CAD build for the part. Positions are in the model's coordinates, mm. Face numbers are marked on the shaded views. A direction names the side the tool comes from. Give positions to 0.01 mm unless a question says otherwise; leave off trailing zeros. Loops run counter-clockwise (first coordinate to the right, second up) from the corner with the lowest first, then second, coordinate; pieces in that order, holes last. Notation, with made-up numbers: (67, 81) - (123, 81) arc R25 cw to (123, 105) - close; hole circle Ø7 at (32, -29). An arc over 180 degrees is marked (long way). Return JSON: item names as keys, results as strings.
from build123d import *

# Parameters (mm, degrees)
BOSS_EXTRUDE2_DEPTH = 80
SKETCH3_R           = 2
CUT_EXTRUDE2_DEPTH  = 80
SKETCH4_W           = 20
SKETCH4_H           = 80
BOSS_EXTRUDE3_DEPTH = 50
BOSS_EXTRUDE4_DEPTH = 80
SKETCH6_W           = 12
SKETCH6_H           = 60
CUT_EXTRUDE4_DEPTH  = 90
SKETCH7_W           = 3
SKETCH7_H           = 68
CUT_EXTRUDE5_DEPTH  = 90
SKETCH9_R           = 2
CUT_EXTRUDE6_DEPTH  = 90
SKETCH11_R          = 2
CUT_EXTRUDE7_DEPTH  = 90


with BuildPart() as part:
    # Sketch1 → Boss-Extrude2 (new body)
    with BuildSketch(Plane.XY):
        with BuildLine():
            ThreePointArc((26, -15.25), (25.707106781, -15.957106781), (25, -16.25))
            Line((25, -16.25), (-19, -16.25))
            Line((-19, -16.25), (-19, 16.25))
            Line((-19, 16.25), (4, 16.25))
            Line((4, 16.25), (53, 16.25))
            ThreePointArc((53, 16.25), (53.707106781, 15.957106781), (54, 15.25))
            Line((54, 15.25), (54, 10.25))
            Line((54, 10.25), (2, 10.25))
            ThreePointArc((2, 10.25), (0.585786438, 9.664213562), (0, 8.25))
            Line((0, 8.25), (0, -8.25))
            ThreePointArc((0, -8.25), (0.585786438, -9.664213562), (2, -10.25))
            Line((2, -10.25), (25, -10.25))
            ThreePointArc((25, -10.25), (25.707106781, -10.542893219), (26, -11.25))
            Line((26, -11.25), (26, -15.25))
        make_face()
    extrude(amount=BOSS_EXTRUDE2_DEPTH)

    # Sketch3 → Cut-Extrude2 (cut)
    with BuildSketch(Plane(origin=(0, 16.25, 0), x_dir=(1, 0, 0), z_dir=(0, 1, 0))):
        with Locations(Location((10.2, -40, 0), (0, 0, 270))):
            Circle(SKETCH3_R)
        with Locations(Location((10.2, -60, 0), (0, 0, 270))):
            Circle(SKETCH3_R)
        with Locations(Location((10.2, -20, 0), (0, 0, 270))):
            Circle(SKETCH3_R)
    extrude(amount=-CUT_EXTRUDE2_DEPTH, mode=Mode.SUBTRACT)

    # Sketch4 → Boss-Extrude3 (add)
    with BuildSketch(Plane(origin=(0, 16.25, 0), x_dir=(1, 0, 0), z_dir=(0, 1, 0))):
        with Locations((-9, -40)):
            Rectangle(SKETCH4_W, SKETCH4_H)
    extrude(amount=BOSS_EXTRUDE3_DEPTH)

    # Sketch5 → Boss-Extrude4 (add)
    with BuildSketch(Plane.XY.offset(80)):
        with BuildLine():
            ThreePointArc((4.354101966, 16.25), (2.2624519, 16.94375696), (1, 18.75))
            Line((1, 18.75), (1, 16.25))
            Line((1, 16.25), (4.354101966, 16.25))
        make_face()
    extrude(amount=-BOSS_EXTRUDE4_DEPTH)

    # Sketch6 → Cut-Extrude4 (cut)
    with BuildSketch(Plane(origin=(0, 66.25, 0), x_dir=(1, 0, 0), z_dir=(0, 1, 0))):
        with Locations((-13, -40)):
            Rectangle(SKETCH6_W, SKETCH6_H)
        with BuildLine():
            ThreePointArc((-17.5, -80), (-18.560660172, -79.560660172), (-19, -78.5))
            Line((-19, -78.5), (-19, -80))
            Line((-19, -80), (-17.5, -80))
        make_face()
        with BuildLine():
            Line((-19, 0), (-19, -1.5))
            ThreePointArc((-19, -1.5), (-18.560660172, -0.439339828), (-17.5, 0))
            Line((-17.5, 0), (-19, 0))
        make_face()
    extrude(amount=-CUT_EXTRUDE4_DEPTH, mode=Mode.SUBTRACT)

    # Sketch7 → Cut-Extrude5 (cut)
    with BuildSketch(Plane(origin=(0, 66.25, 0), x_dir=(1, 0, 0), z_dir=(0, 1, 0))):
        with Locations((-8.5, -40)):
            Rectangle(SKETCH7_W, SKETCH7_H)
    extrude(amount=-CUT_EXTRUDE5_DEPTH, mode=Mode.SUBTRACT)

    # Sketch9 → Cut-Extrude6 (cut)
    with BuildSketch(Plane(origin=(1, 0, 0), x_dir=(0, 0, -1), z_dir=(1, 0, 0))):
        with Locations(Location((-49.9, 36.25, 0), (0, 0, 90))):
            Circle(SKETCH9_R)
        with Locations(Location((-30.1, 36.25, 0), (0, 0, 90))):
            Circle(SKETCH9_R)
    extrude(amount=-CUT_EXTRUDE6_DEPTH, mode=Mode.SUBTRACT)

    # Sketch11 → Cut-Extrude7 (cut)
    with BuildSketch(Plane(origin=(1, 0, 0), x_dir=(0, 0, -1), z_dir=(1, 0, 0))):
        with Locations(Location((-40, 36.25, 0), (0, 0, 90))):
            Circle(SKETCH11_R)
    extrude(amount=-CUT_EXTRUDE7_DEPTH, mode=Mode.SUBTRACT)


solid = part.part
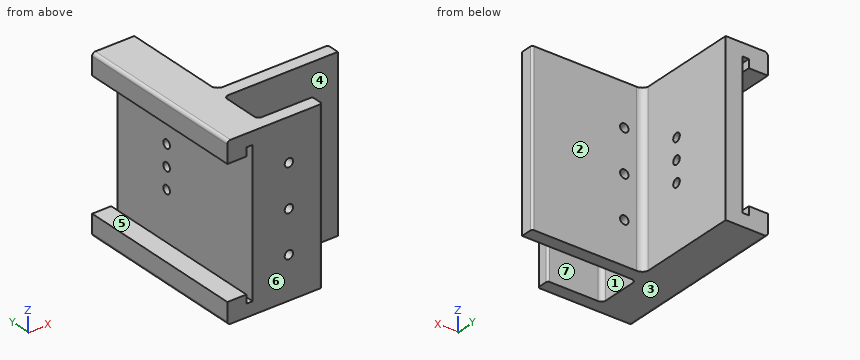
1. Drill centre lines: probe 1 along Z at (x, y) = (10, -12); probe 2 along Z at (x, y) = (-0.75, 36.25); probe 3 along Y at (x, z) = (20, 76.5). Where is each one in solid material? Low to high.
Values follow:
{"probe 1": "z = 0 to 18.01, 21.99 to 38.01, 41.99 to 58.01, 61.99 to 80", "probe 2": "z = 0 to 28.1, 32.1 to 38, 42 to 47.9, 51.9 to 80", "probe 3": "y = -16.25 to -10.25, 10.25 to 16.25"}
2. Which spindle directions (+Z, -Z, +X, -X, +Y, -Y) get a long thin tool onto all of the face, cutting with end or side? Do the marked faces 1, 2 and 3. Say none if no direction does.
Values follow:
{"face 1": "+Z, -Z, +X", "face 2": "+Z, -Z, +X, +Y", "face 3": "-Z, +X, -X, +Y, -Y"}
3. Cut at C-C, the plane x = 10.2. Give the number of separate pieces and of enclosed holes in the cut face, plus the area to 3 significant figures.
Values follow:
{"separate pieces": "8", "enclosed holes": "0", "area": "816 mm²"}
4. Cut at B-B, the plane y = 36.25. Write the cut outline in (x, z).
Values follow:
{"outline": "(-19, 1.5) arc R1.5 ccw to (-17.5, 0) - (1, 0) - (1, 28.1) - (-7, 28.1) - (-7, 6) - (-10, 6) - (-10, 10) - (-19, 10) - close; (-19, 70) - (-10, 70) - (-10, 74) - (-7, 74) - (-7, 51.9) - (1, 51.9) - (1, 80) - (-17.5, 80) arc R1.5 ccw to (-19, 78.5) - close; (-7, 32.1) - (1, 32.1) - (1, 38) - (-7, 38) - close; (-7, 42) - (1, 42) - (1, 47.9) - (-7, 47.9) - close"}
5. Pull direction Y, two halves, no side cores. Call the marked faces 4, 5, 6 and 7: +Y half, -Y half, draft (parallel to the pull), parting line (faces both ways), or undercut.
Values follow:
{"face 4": "undercut", "face 5": "draft", "face 6": "-Y half", "face 7": "undercut"}
6. Cut at D-D, the plane z = 30.1. Write the cut outline in (x, y), plus the area to 3 significant figures.
Values follow:
{"outline": "(-7, -16.25) - (25, -16.25) arc R1 ccw to (26, -15.25) - (26, -11.25) arc R1 ccw to (25, -10.25) - (2, -10.25) arc R2 cw to (0, -8.25) - (0, 8.25) arc R2 cw to (2, 10.25) - (54, 10.25) - (54, 15.25) arc R1 ccw to (53, 16.25) - (4.35, 16.25) arc R3.5 cw to (1, 18.75) - (1, 34.25) - (-7, 34.25) - close; (-7, 38.25) - (1, 38.25) - (1, 66.25) - (-7, 66.25) - close", "area": "1,080 mm²"}
7. Cut at A-A, the plane z = 20. Write the cut outline in (x, y), plus the area to 3 significant figures.
Values follow:
{"outline": "(-7, -16.25) - (8.2, -16.25) - (8.2, -10.25) - (2, -10.25) arc R2 cw to (0, -8.25) - (0, 8.25) arc R2 cw to (2, 10.25) - (8.2, 10.25) - (8.2, 16.25) - (4.35, 16.25) arc R3.5 cw to (1, 18.75) - (1, 66.25) - (-7, 66.25) - close; (12.2, -16.25) - (25, -16.25) arc R1 ccw to (26, -15.25) - (26, -11.25) arc R1 ccw to (25, -10.25) - (12.2, -10.25) - close; (12.2, 10.25) - (54, 10.25) - (54, 15.25) arc R1 ccw to (53, 16.25) - (12.2, 16.25) - close", "area": "1,060 mm²"}
8. Drop flat-ended pins along their axis: P1, Ø24, axis at y = 48.5, z = 57, coming from the +X side; P2, Ø5, axis at x = 30.5, z = 23, coming from the +Y side; P3, Ø8, axis at y = 4, z = 52.5, coming from the +X side. Give the stop position or say it passes through.
Values follow:
{"P1": "stops at x = 1", "P2": "stops at y = 16.25", "P3": "stops at x = 0"}
